Geometry check sheet. Reference: drawing and pictorial views, mm from the part's lowest x, y, z. A direction names the side the tool comes from. Give positions to 0.01 mm unless a question says otherwise; leave off trailing zeros. Write each loop counter-clockwise with the first axis right and the second up, starting at its lowest first coordinate (ties: lowest second). Pieces come first, ordered by that corner, then holes.
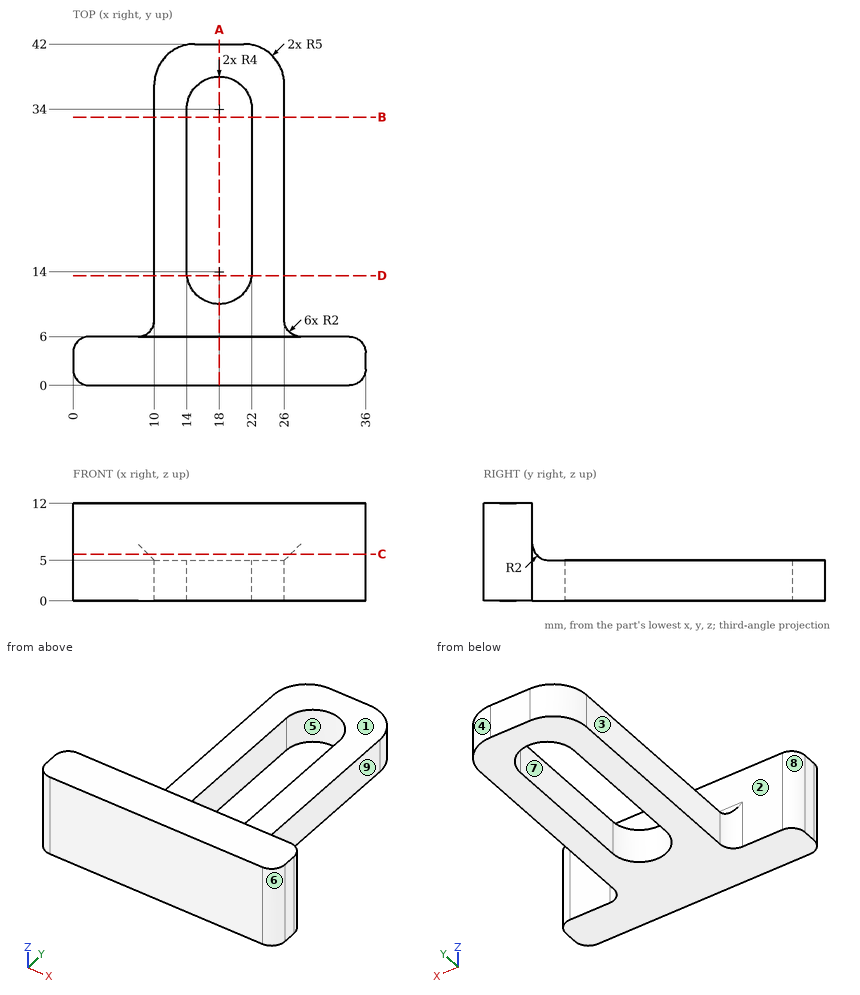
Item 1: Sectioned sample at A-A on x = 18. Record the cut outline in (y, z), then the cut area to 3 significant figures.
Answer key:
outline: (0, 0) - (10, 0) - (10, 5) - (8, 5) arc R2 cw to (6, 7) - (6, 12) - (0, 12) - close; (38, 0) - (42, 0) - (42, 5) - (38, 5) - close
area: 113 mm2
Item 2: Sectioned sample at D-D on y = 13.5. Record the cut outline in (x, z).
Answer key:
outline: (10, 0) - (14.03, 0) - (14.03, 5) - (10, 5) - close; (21.97, 0) - (26, 0) - (26, 5) - (21.97, 5) - close
Item 3: Set-up check for the marked faces 1, 2, 3, 4 and 5: record each of +Z, -Z, +X, -X, +Y, -Y from which the full face is reachable in a straight line by a thin tool's end or side.
Answer key:
face 1: +Z, +X, -X, +Y
face 2: +Z, +Y
face 3: +Z, -Z, -X, +Y
face 4: +Z, -Z, +X, +Y
face 5: +Z, -Z
Item 4: Depth check by flat-ended pin: pin 1 (12 mm diameter, centred on x = 8, y = 37, fed in from -Z); pin 2 (1 mm diameter, centred on x = 19, z = 10, fed in from +Y); pin 3 (1.5 mm diameter, centred on y = 23.5, z = 3, fed in from +X); pin 4 (3 mm diameter, centred on y = 7, z = 9.5, fed in from -X). Enter the tip coordinate at first touch or a pass-through.
Answer key:
pin 1: stops at z = 0
pin 2: stops at y = 6
pin 3: stops at x = 26
pin 4: stops at x = 0.68
Item 5: Scan lines: line 1 along X through (y, z) = (23.5, 3); line 2 along Y through (x, z) = (22, 7.5); line 3 along Z through (x, y) = (25, 14). Record each from-to range of solid material in increasing order.
Answer key:
line 1: x = 10 to 14, 22 to 26
line 2: y = 0 to 6
line 3: z = 0 to 5
Item 6: Sectioned sample at B-B on y = 33. Record the cut outline in (x, z).
Answer key:
outline: (10, 0) - (14, 0) - (14, 5) - (10, 5) - close; (22, 0) - (26, 0) - (26, 5) - (22, 5) - close
Item 7: Sectioned sample at C-C on z = 5.75. Record the cut outline in (x, y), then the cut area to 3 significant figures.
Answer key:
outline: (0, 2) arc R2 ccw to (2, 0) - (34, 0) arc R2 ccw to (36, 2) - (36, 4) arc R2 ccw to (34, 6) - (28, 6) arc R2 cw to (26.75, 6.44) - (9.25, 6.44) arc R2 cw to (8, 6) - (2, 6) arc R2 ccw to (0, 4) - close
area: 221 mm2
Item 8: Release check for a two-part mould opening along Y. For the marked faces 6, 7, 8 and 9 record: released by +Y, released by -Y, zero draft, split by the parting line, or undercut.
Answer key:
face 6: released by -Y
face 7: undercut
face 8: released by +Y
face 9: zero draft
